from build123d import *

# Parameters (mm, degrees)
ESQUISSE1_W                 = 33
ESQUISSE1_H                 = 10
ESQUISSE1_R                 = 1
EXTRUSION1_DEPTH            = 1.5
ENL_V_START                 = -1.5
ENL_V_MAT_EXTRU_1_OUTLINE_R = 1
ENL_V_MAT_EXTRU_1_DEPTH     = 1.5


# Read off the part's stored shape, not the designer's step: Enlèv. mat.-Extru.1
with BuildPart() as part:
    # Esquisse1 → Extrusion1 (new body)
    with BuildSketch(Plane(origin=(0, 0, 0), x_dir=(1, 0, 0), z_dir=(0, 1, 0))):
        with Locations((29.365732097, 0)):
            Rectangle(ESQUISSE1_W, ESQUISSE1_H)
        with Locations(Location((42.865732097, 0, 0), (0, 0, 270))):
            Circle(ESQUISSE1_R, mode=Mode.SUBTRACT)
        with Locations(Location((15.865732097, 0, 0), (0, 0, 270))):
            Circle(ESQUISSE1_R, mode=Mode.SUBTRACT)
        Polygon((36.878065896, 3.001382291), (36.86981937, 3.101041684), (38.065732097, 3.2), (38.073978624, 3.100340606), align=None, mode=Mode.SUBTRACT)
        Polygon((34.328504824, 2.890755264), (34.33675135, 2.79109587), (35.532664078, 2.890054186), (35.524417551, 2.989713579), align=None, mode=Mode.SUBTRACT)
        Polygon((31.787190278, 2.680468843), (31.795436804, 2.580809449), (32.991349532, 2.679767765), (32.983103005, 2.779427159), align=None, mode=Mode.SUBTRACT)
        Polygon((29.245875732, 2.470182423), (29.254122258, 2.370523029), (30.450034986, 2.469481345), (30.44178846, 2.569140738), align=None, mode=Mode.SUBTRACT)
        Polygon((26.704561186, 2.259896002), (26.712807712, 2.160236608), (27.90872044, 2.259194924), (27.900473914, 2.358854318), align=None, mode=Mode.SUBTRACT)
        Polygon((24.16324664, 2.049609582), (24.171493166, 1.949950188), (25.367405894, 2.048908503), (25.359159368, 2.148567897), align=None, mode=Mode.SUBTRACT)
        Polygon((21.621932094, 1.839323161), (21.630178621, 1.739663767), (22.826091348, 1.838622083), (22.817844822, 1.938281477), align=None, mode=Mode.SUBTRACT)
        Polygon((19.080617548, 1.629036741), (19.088864075, 1.529377347), (20.284776802, 1.628335662), (20.276530276, 1.727995056), align=None, mode=Mode.SUBTRACT)
        Polygon((22.294666135, -1.894989955), (22.302912661, -1.795330561), (23.498825389, -1.894288877), (23.490578862, -1.993948271), align=None, mode=Mode.SUBTRACT)
        Polygon((27.377295227, -2.315562796), (27.385541753, -2.215903402), (28.581454481, -2.314861718), (28.573207954, -2.414521112), align=None, mode=Mode.SUBTRACT)
        Polygon((32.459924319, -2.736135637), (32.468170845, -2.636476244), (33.664083572, -2.735434559), (33.655837046, -2.835093953), align=None, mode=Mode.SUBTRACT)
        Polygon((35.001238865, -2.946422058), (35.009485391, -2.846762664), (36.205398118, -2.94572098), (36.197151592, -3.045380374), align=None, mode=Mode.SUBTRACT)
        Polygon((29.918609773, -2.525849217), (29.926856299, -2.426189823), (31.122769027, -2.525148139), (31.1145225, -2.624807532), align=None, mode=Mode.SUBTRACT)
        Polygon((24.835980681, -2.105276376), (24.844227207, -2.005616982), (26.040139935, -2.104575297), (26.031893408, -2.204234691), align=None, mode=Mode.SUBTRACT)
        Polygon((19.753351589, -1.684703535), (19.761598115, -1.585044141), (20.957510843, -1.684002456), (20.949264317, -1.78366185), align=None, mode=Mode.SUBTRACT)
    extrude(amount=-EXTRUSION1_DEPTH)

    # Enlèv. mat.-Extru.1 outline → Enlèv. mat.-Extru.1 (cut)
    # profile 1 of 2: a face of its own
    with BuildSketch(Plane(origin=(0, 0, 0), x_dir=(1, 0, 0), z_dir=(0, 1, 0)).offset(ENL_V_START)):
        Polygon((24.723817468, -4.419702073), (22.083186059, 5), (12.865732097, 5), (12.865732097, -5), (24.397634062, -5), align=None)
        Polygon((20.949264317, -1.78366185), (19.753351589, -1.684703535), (19.761598115, -1.585044141), (20.957510843, -1.684002456), align=None, mode=Mode.SUBTRACT)
        Polygon((23.490578862, -1.993948271), (22.294666135, -1.894989955), (22.302912661, -1.795330561), (23.498825389, -1.894288877), align=None, mode=Mode.SUBTRACT)
        with Locations((15.865732097, 0)):
            Circle(ENL_V_MAT_EXTRU_1_OUTLINE_R, mode=Mode.SUBTRACT)
        Polygon((19.080617548, 1.629036741), (20.276530276, 1.727995056), (20.284776802, 1.628335662), (19.088864075, 1.529377347), align=None, mode=Mode.SUBTRACT)
        Polygon((21.621932094, 1.839323161), (22.817844822, 1.938281477), (22.826091348, 1.838622083), (21.630178621, 1.739663767), align=None, mode=Mode.SUBTRACT)
    # profile 2 of 2: a face of its own
    with BuildSketch(Plane(origin=(0, 0, 0), x_dir=(1, 0, 0), z_dir=(0, 1, 0)).offset(ENL_V_START)):
        Polygon((45.865732097, 5), (39.738529372, 5), (42.541836089, -5), (45.865732097, -5), align=None)
        with Locations((42.865732097, 0)):
            Circle(ENL_V_MAT_EXTRU_1_OUTLINE_R, mode=Mode.SUBTRACT)
    extrude(amount=ENL_V_MAT_EXTRU_1_DEPTH, mode=Mode.SUBTRACT)


solid = part.part
Work out the finished part from the listing and answer in its coordinate system (mm). Coordinates: 2 decimals unless noted, no trailing zeros. Loops run counter-clockwise (first coordinate to the right, second up) from the corner with the lowest first, then second, coordinate; pieces in that order, holes last. Notation, with made-up numbers: M 5.5,47.25 L 28.5,47.25 A27 ccw 28.5,63.25 Z; hole C 81,-21 d10. An arc over 180 degrees is marked long. Answer in a Markdown table with one row per item. Add a question column.
1. Find section B-B, the plane z = 0.25. Write down the section's boundary in (x, y).
2. Consider L1, parallel to X at y = -0.85, z = -4.5; L2, parallel to X at y = -1.3, z = 4.25. Determine where each line is inside the solid, lowest interval first.
3. Find section C-C, the plane x = 41. Write down the section's boundary in (y, z), then the cut area to 3 significant figures.
4. Find section A-A, the plane y = -0.2. State how many separate pieces and enclosed holes the cut face has, then the cut area to 3 significant figures.
Reported:
| question | item | result |
|---|---|---|
| 1 | outline | M 23.55,-1.5 L 41.21,-1.5 L 41.21,0 L 23.55,0 Z |
| 2 | L1 | x = 22.22 to 39.88 |
| 2 | L2 | x = 24.68 to 42.33 |
| 3 | outline | M -1.5,-0.5 L 0,-0.5 L 0,5 L -1.5,5 Z |
| 3 | area | 8.25 mm^2 |
| 4 | separate pieces | 1 |
| 4 | enclosed holes | 11 |
| 4 | area | 175 mm^2 |
